Design review of the part shown in the three views and the two pictorial views. Dimensions are in mm from the part's minimum x, y and z. Give positions to 0.01 mm unless a question says otherwise; leave off trailing zeros. Loops run counter-clockwise (first coordinate to the right, second up) from the corner with the lowest first, then second, coordinate; pieces in that order, holes last. Notation, with made-up numbers: (8.5, -13) - (64.5, -13) arc R25 cw to (64.5, 21) - close; hole circle Ø6 at (-15.75, -32.75). An arc over 180 degrees is marked (long way). Use CSV: the item, a comma, the result in double quotes. Start each with the question number.
1. For pin 1 (2 mm diameter, centred on x = 27, z = 23.5, fed in from -Y); pin 2 (1.5 mm diameter, centred on x = 7, z = 54.5, fed in from -Y), all flat-tipped, find the tip position at first contact; note any pin that passes through.
2. Take a section at B-B on x = 8.5. Give the boundary of the cut face in (y, z), plus the area to 3 significant figures.
3. Mouldability with a two-part tool opening along X and no side actions: class the marked faces 1, 2 and 3 as pulls with the +X half, pulls with the -X half, needs draft (parallel to the pull), parting line crosses it, or undercut.
4. Wall thickness on line 1 (X direction, y = 4.25, z = 45.5); line 2 (X direction, y = 2.5, z = 12.5); line 3 (Y direction, x = 9, z = 43): over which ranges is each line inside the solid? List them lowest first.
5. Take a section at A-A on z = 34.5. Give the boundary of the cut face in (x, y).
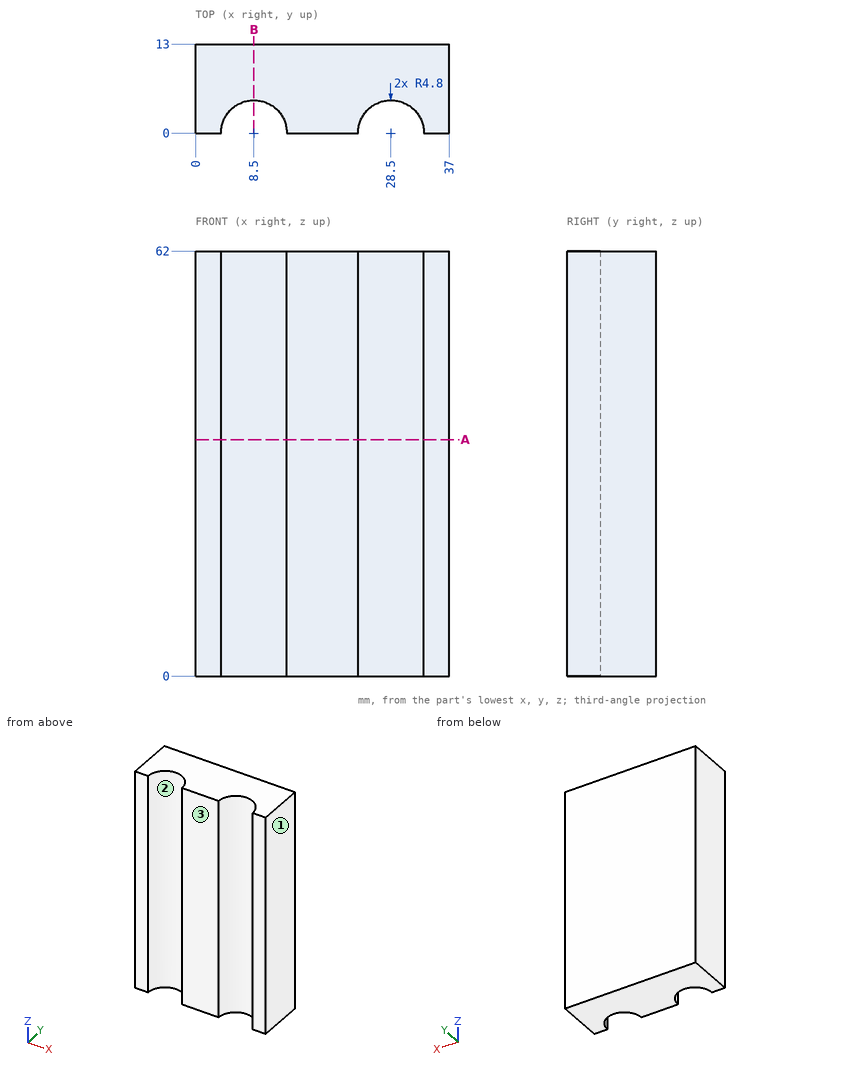
Check result:
1,pin 1,"stops at y = 4.1"
1,pin 2,"stops at y = 4.24"
2,outline,"(4.8, 0) - (13, 0) - (13, 62) - (4.8, 62) - close"
2,area,"508 mm²"
3,face 1,"pulls with the +X half"
3,face 2,"undercut"
3,face 3,"needs draft"
4,line 1,"x = 0 to 6.27, 10.73 to 26.27, 30.73 to 37"
4,line 2,"x = 0 to 4.4, 12.6 to 24.4, 32.6 to 37"
4,line 3,"y = 4.77 to 13"
5,outline,"(0, 0) - (3.7, 0) arc R4.8 cw to (13.3, 0) - (23.7, 0) arc R4.8 cw to (33.3, 0) - (37, 0) - (37, 13) - (0, 13) - close"
